The listing builds one solid part. Answer for the finished solid, in the listing's coordinates (mm). A direction names the side the tool comes from. Coordinates: 2 decimals unless noted, no trailing zeros. Order: outer loops, then holes, each group sorted by start corner. A loop starts at its lowest first (then second) coordinate and runs counter-clockwise, first axis right, second up.
from build123d import *

# Parameters (mm, degrees)
BOSS_EXTRU_2_DEPTH        = 6.35
ESQUISSE29_R              = 6
BOSS_EXTRU_3_DEPTH        = 6.35
SYM_TRIE2_COPY_1_SKETCH_R = 6
SYM_TRIE2_COPY_1_DEPTH    = 6.35
ESQUISSE30_R              = 2
ENL_V_MAT_EXTRU_1_DEPTH   = 48.7671004
CONG_1_R                  = 5


with BuildPart() as part:
    # Esquisse28 → Boss.-Extru.2 (new body)
    with BuildSketch(Plane.XY):
        Polygon((-21.5, -28.005382387), (-28.005382387, -21.5), (-28.005382387, 21.5), (-21.5, 28.005382387), (21.5, 28.005382387), (28.005382387, 21.5), (28.005382387, -21.5), (21.5, -28.005382387), align=None)
        Polygon((-16.978069991, -21.15), (-21.15, -16.978069991), (-21.15, 16.978069991), (-16.978069991, 21.15), (16.978069991, 21.15), (21.15, 16.978069991), (21.15, -16.978069991), (16.978069991, -21.15), align=None, mode=Mode.SUBTRACT)
    extrude(amount=BOSS_EXTRU_2_DEPTH)

    # Esquisse29 → Boss.-Extru.3 (add)
    with BuildSketch(Plane.XY):
        with Locations((27.476658888, 27.476658888)):
            Circle(ESQUISSE29_R)
    boss_extru_3 = extrude(amount=BOSS_EXTRU_3_DEPTH)

    # Symétrie1: Boss.-Extru.3 across plane
    add(boss_extru_3.mirror(Plane(origin=(0, 0, 0), x_dir=(0, 0, 1), z_dir=(1, 0, 0))))

    # Symétrie2: Boss.-Extru.3 across plane
    add(boss_extru_3.mirror(Plane.ZX))

    # Symétrie2 copy 1 sketch → Symétrie2 copy 1 (add)
    with BuildSketch(Plane(origin=(0, 0, 0), x_dir=(-1, 0, 0), z_dir=(0, 0, 1))):
        with Locations((27.476658888, 27.476658888)):
            Circle(SYM_TRIE2_COPY_1_SKETCH_R)
    extrude(amount=SYM_TRIE2_COPY_1_DEPTH)

    # Esquisse30 → Enlèv. mat.-Extru.1 (cut, through all)
    with BuildSketch(Plane.XY.offset(6.35)):
        with Locations((-27.476658888, 27.476658888)):
            Circle(ESQUISSE30_R)
        with Locations((27.476658888, 27.476658888)):
            Circle(ESQUISSE30_R)
        with Locations((27.476658888, -27.476658888)):
            Circle(ESQUISSE30_R)
        with Locations((-27.476658888, -27.476658888)):
            Circle(ESQUISSE30_R)
    extrude(amount=-ENL_V_MAT_EXTRU_1_DEPTH, mode=Mode.SUBTRACT)

    # Congé1
    cong_1_edges = [part.edges().sort_by_distance(p)[0] for p in [
        (-21.5, -28.005382387, 3.175),
        (-28.005382387, -21.5, 3.175),
        (-28.005382387, 21.5, 3.175),
        (-21.5, 28.005382387, 3.175),
        (21.5, 28.005382387, 3.175),
        (28.005382387, 21.5, 3.175),
        (28.005382387, -21.5, 3.175),
        (21.5, -28.005382387, 3.175),
    ]]
    fillet(cong_1_edges, radius=CONG_1_R)


solid = part.part
1) Determine the mould class of faces 5 (the face through (-26.55, -29.25, 3.22)), 6 (the face through (0, -28.005, 3)), 7 (the face through (20.429, 28.653, 3.219)), 8 (the face through (0, 22, 0)) for opening direction Y: released by +Y, released by -Y, zero draft, split by the parting line, or undercut.
2) Section A-A (y = -10) is taken. Give the vertices of the cut face in (x, z), then the cut area to 3 significant figures.
3) Consider L1, parallel to X at y = 6.5, z = 0.5; L2, parallel to Y at x = 29, z = 2.5. Determine where each line is inside the solid, lowest interval first.
4) Section D-D (z = 3.5) is taken. Give the vertices of the cut face in (x, y), then the cut area to 3 significant figures.
5) Section C-C (x = 27) is taken. Give the vertices of the cut face in (y, z).
6) A tool of negligible diameter and unlimited length cuts with its end or side. For faces 1 (the face through (28.653, 20.429, 3.219)), 2 (the face through (-20.49, -28.69, 3.22)), 3 (the face through (-28.69, -20.49, 3.22)), 4 (the face through (0, 21.15, 3)), from which of +Z, -Z, +X, -X, +Y, -Y can it reach the whole face along a straight path? Write none if from no direction.
7) Each of these flat-tipped pins is pushed along its axis until it touches: P1, Ø1.9, axis at y = 5.5, z = 2, coming from the +X side; P2, Ø6.5, axis at x = -27.48, y = 27.48, coming from the +Z side; P3, Ø1.9, axis at y = -2, z = 3, coming from the -X side; P4, Ø1, axis at x = 3, z = 1.5, coming from the +Y side. Where does it stop, or does it pass through?
Filled sheet:
1. face 5: undercut
1. face 6: released by -Y
1. face 7: released by +Y
1. face 8: zero draft
2. outline: (-28.01, 0) - (-21.15, 0) - (-21.15, 6.35) - (-28.01, 6.35) - close; (21.15, 0) - (28.01, 0) - (28.01, 6.35) - (21.15, 6.35) - close
2. area: 87.1 mm2
3. L1: x = -28.01 to -21.15, 21.15 to 28.01
3. L2: y = -33.28 to -28.77, -26.18 to -20.96, 20.96 to 26.18, 28.77 to 33.28
4. outline: (-30.49, -22.29) arc R6 ccw (long way) to (-22.29, -30.49) arc R5 cw to (-17.97, -28.01) - (17.97, -28.01) arc R5 cw to (22.29, -30.49) arc R6 ccw (long way) to (30.49, -22.29) arc R5 cw to (28.01, -17.97) - (28.01, 17.97) arc R5 cw to (30.49, 22.29) arc R6 ccw (long way) to (22.29, 30.49) arc R5 cw to (17.97, 28.01) - (-17.97, 28.01) arc R5 cw to (-22.29, 30.49) arc R6 ccw (long way) to (-30.49, 22.29) arc R5 cw to (-28.01, 17.97) - (-28.01, -17.97) arc R5 cw to start; hole circle Ø4 at (-27.48, -27.48); hole circle Ø4 at (-27.48, 27.48); hole (-21.15, -16.98) - (-16.98, -21.15) - (16.98, -21.15) - (21.15, -16.98) - (21.15, 16.98) - (16.98, 21.15) - (-16.98, 21.15) - (-21.15, 16.98) - close; hole circle Ø4 at (27.48, -27.48); hole circle Ø4 at (27.48, 27.48)
4. area: 1,660 mm2
5. outline: (-33.46, 0) - (-29.42, 0) - (-29.42, 6.35) - (-33.46, 6.35) - close; (-25.53, 0) - (25.53, 0) - (25.53, 6.35) - (-25.53, 6.35) - close; (29.42, 0) - (33.46, 0) - (33.46, 6.35) - (29.42, 6.35) - close
6. face 1: +Z, -Z, +X
6. face 2: +Z, -Z, -Y
6. face 3: +Z, -Z, -X
6. face 4: +Z, -Z
7. P1: stops at x = 28.01
7. P2: stops at z = 6.35
7. P3: stops at x = -28.01
7. P4: stops at y = 28.01
